Verification items for the finished model (mm, model axes). Face numbers are marked on the shaded views. A direction names the side the tool comes from. Give positions to 0.01 mm unless a question says otherwise; leave off trailing zeros. Loops run counter-clockwise (first coordinate to the right, second up) from the corner with the lowest first, then second, coordinate; pieces in that order, holes last. Notation, with made-up numbers: M 11.25,-28 L 70.25,-28 A9 cw 70.25,-11 Z; hole C -34.5,-14.5 d1. An arc over 180 degrees is marked long. Put each result on its own line as item: value. Start each with the question number.
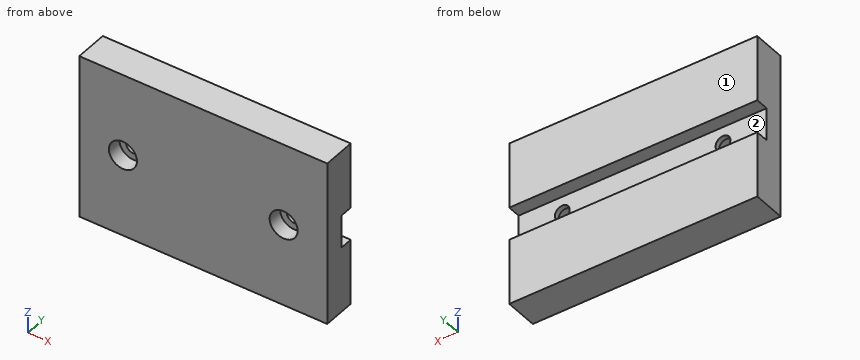
from build123d import *

# Parameters (mm, degrees)
F0_W           = 75.186654
F0_H           = 50
F1_DEPTH       = 10
F2_W           = 4
F2_H           = 10
F3_DEPTH       = 75.187655
F5_D           = 4.5
F5_CBORE_D     = 8.5
F5_CBORE_DEPTH = 4.5


with BuildPart() as f1:
    # F0 (on Front) → F1 (new body)
    with BuildSketch(Plane.XZ):
        Rectangle(F0_W, F0_H)
    extrude(amount=F1_DEPTH)

    # F2 (on face) → F3 (cut, through all)
    with BuildSketch(Plane.YZ.offset(37.593327)):
        with Locations((-2, 0)):
            Rectangle(F2_W, F2_H)
    extrude(amount=-F3_DEPTH, mode=Mode.SUBTRACT)

    # F5 (through all)
    with Locations(Plane.XZ.offset(10)):
        with Locations((-24.358043, 0), (24.358043, 0)):
            CounterBoreHole(F5_D / 2, F5_CBORE_D / 2, F5_CBORE_DEPTH)


solid = f1.part
Q1. Set-up check for the marked faces 1 and 2: record each of +Z, -Z, +X, -X, +Y, -Y from which the full face is reachable in a straight line by a thin tool's end or side.
Q2. Scan lines: L1, parallel to Z at x = 10.5, y = -1; L2, parallel to Y at x = -18, z = 2; L3, parallel to X at y = -6.25, z = 3. Record each from-to range of solid material in increasing order.
Q3. Cross-section at C-C, the plane x = 5. Record the boundary of the cut face in (y, z), then the cut area to 3 significant figures.
Q4. Cross-section at A-A, the plane y = -1.5. Record the boundary of the cut face in (x, z).
Q5. Go/stop test with flat-tipped pins: pin 1 (7 mm diameter, centred on x = -24.36, z = 0, fed in from -Y); pin 2 (7 mm diameter, centred on x = -24.36, z = 0, fed in from +Y); pin 3 (4 mm diameter, centred on x = 24.36, z = 0, fed in from -Y). Record where each tip stops, or that it passes through.
Q6. Cross-section at B-B, the plane z = 0. Record the boundary of the cut face in (x, y).
Q7. Cross-section at D-D, the plane x = 24.5. Record the boundary of the cut face in (y, z), then the cut area to 3 significant figures.
Ans:
1. face 1: +Z, -Z, +X, -X, +Y
1. face 2: +X, -X, +Y
2. L1: z = -25 to -5, 5 to 25
2. L2: y = -10 to -4
2. L3: x = -37.59 to -27.37, -21.35 to 21.35, 27.37 to 37.59
3. outline: M -10,-25 L 0,-25 L 0,-5 L -4,-5 L -4,5 L 0,5 L 0,25 L -10,25 Z
3. area: 460 mm^2
4. outline: M -37.59,-25 L 37.59,-25 L 37.59,-5 L -37.59,-5 Z; M -37.59,5 L 37.59,5 L 37.59,25 L -37.59,25 Z
5. pin 1: stops at y = -5.5
5. pin 2: stops at y = -4
5. pin 3: passes through
6. outline: M -37.59,-10 L -28.61,-10 L -28.61,-5.5 L -26.61,-5.5 L -26.61,-4 L -37.59,-4 Z; M -22.11,-5.5 L -20.11,-5.5 L -20.11,-10 L 20.11,-10 L 20.11,-5.5 L 22.11,-5.5 L 22.11,-4 L -22.11,-4 Z; M 26.61,-5.5 L 28.61,-5.5 L 28.61,-10 L 37.59,-10 L 37.59,-4 L 26.61,-4 Z
7. outline: M -10,-25 L 0,-25 L 0,-5 L -4,-5 L -4,-2.25 L -5.5,-2.25 L -5.5,-4.25 L -10,-4.25 Z; M -10,4.25 L -5.5,4.25 L -5.5,2.25 L -4,2.25 L -4,5 L 0,5 L 0,25 L -10,25 Z
7. area: 415 mm^2
